Design review of the part built by this model. Coordinates are the model's own, in mm. Face numbers are marked on the shaded views. Coordinates: 2 decimals unless noted, no trailing zeros. Write each loop counter-clockwise with the first axis right and the second up, starting at its lowest first coordinate (ties: lowest second). Pieces come first, ordered by that corner, then holes. Notation, with made-up numbers: M 85.5,11 L 106.5,11 A27 ccw 106.5,28 Z; hole C 19,-31.75 d7. An arc over 180 degrees is marked long. Return JSON: item names as keys, results as strings. Group by question number.
```python
from build123d import *

# Parameters (mm, degrees)
SKETCH1_W           = 110
SKETCH1_H           = 135
SKETCH1_W_2         = 100
SKETCH1_H_2         = 125
BOSS_EXTRUDE1_DEPTH = 200
SKETCH2_W           = 110
SKETCH2_H           = 135
BOSS_EXTRUDE2_DEPTH = 5
CUT_EXTRUDE1_DEPTH  = 12
FILLET1_R           = 3


with BuildPart() as part:
    # Sketch1 → Boss-Extrude1 (new body)
    with BuildSketch(Plane(origin=(0, 0, 0), x_dir=(1, 0, 0), z_dir=(0, 1, 0))):
        Rectangle(SKETCH1_W, SKETCH1_H)
        Rectangle(SKETCH1_W_2, SKETCH1_H_2, mode=Mode.SUBTRACT)
    extrude(amount=BOSS_EXTRUDE1_DEPTH)

    # Sketch2 → Boss-Extrude2 (add)
    with BuildSketch(Plane(origin=(0, 200, 0), x_dir=(1, 0, 0), z_dir=(0, 1, 0))):
        Rectangle(SKETCH2_W, SKETCH2_H)
    extrude(amount=BOSS_EXTRUDE2_DEPTH)

    # Sketch3 → Cut-Extrude1 (cut)
    with BuildSketch(Plane.XZ):
        with BuildLine():
            ThreePointArc((1.45, -65), (0, -63.55), (-1.45, -65))
            Line((-1.45, -65), (1.45, -65))
        make_face()
        with BuildLine():
            Line((1.45, -65), (-1.45, -65))
            ThreePointArc((-1.45, -65), (0, -66.45), (1.45, -65))
        make_face()
        with BuildLine():
            ThreePointArc((53.95, -65), (53.525304833, -63.974695167), (52.5, -63.55))
            Line((52.5, -63.55), (52.5, -65))
            Line((52.5, -65), (51.05, -65))
            ThreePointArc((51.05, -65), (52.5, -66.45), (53.95, -65))
        make_face()
        with BuildLine():
            Line((52.5, -65), (52.5, -63.55))
            ThreePointArc((52.5, -63.55), (51.474695167, -63.974695167), (51.05, -65))
            Line((51.05, -65), (52.5, -65))
        make_face()
        with BuildLine():
            ThreePointArc((53.95, 0), (53.525304833, 1.025304833), (52.5, 1.45))
            Line((52.5, 1.45), (52.5, -1.45))
            ThreePointArc((52.5, -1.45), (53.525304833, -1.025304833), (53.95, 0))
        make_face()
        with BuildLine():
            Line((52.5, -1.45), (52.5, 1.45))
            ThreePointArc((52.5, 1.45), (51.05, 0), (52.5, -1.45))
        make_face()
        with BuildLine():
            ThreePointArc((53.95, 65), (52.5, 66.45), (51.05, 65))
            Line((51.05, 65), (52.5, 65))
            Line((52.5, 65), (52.5, 63.55))
            ThreePointArc((52.5, 63.55), (53.525304833, 63.974695167), (53.95, 65))
        make_face()
        with BuildLine():
            Line((52.5, 65), (51.05, 65))
            ThreePointArc((51.05, 65), (51.474695167, 63.974695167), (52.5, 63.55))
            Line((52.5, 63.55), (52.5, 65))
        make_face()
        with BuildLine():
            ThreePointArc((1.45, 65), (0, 66.45), (-1.45, 65))
            Line((-1.45, 65), (1.45, 65))
        make_face()
        with BuildLine():
            Line((1.45, 65), (-1.45, 65))
            ThreePointArc((-1.45, 65), (0, 63.55), (1.45, 65))
        make_face()
        with BuildLine():
            Line((-52.5, 63.55), (-52.5, 65))
            Line((-52.5, 65), (-51.05, 65))
            ThreePointArc((-51.05, 65), (-53.525304833, 66.025304833), (-52.5, 63.55))
        make_face()
        with BuildLine():
            Line((-51.05, 65), (-52.5, 65))
            Line((-52.5, 65), (-52.5, 63.55))
            ThreePointArc((-52.5, 63.55), (-51.474695167, 63.974695167), (-51.05, 65))
        make_face()
        with BuildLine():
            ThreePointArc((-51.05, 0), (-51.474695167, 1.025304833), (-52.5, 1.45))
            Line((-52.5, 1.45), (-52.5, -1.45))
            ThreePointArc((-52.5, -1.45), (-51.474695167, -1.025304833), (-51.05, 0))
        make_face()
        with BuildLine():
            Line((-52.5, -1.45), (-52.5, 1.45))
            ThreePointArc((-52.5, 1.45), (-53.95, 0), (-52.5, -1.45))
        make_face()
        with BuildLine():
            ThreePointArc((-51.05, -65), (-51.474695167, -63.974695167), (-52.5, -63.55))
            Line((-52.5, -63.55), (-52.5, -65))
            Line((-52.5, -65), (-51.05, -65))
        make_face()
        with BuildLine():
            Line((-52.5, -65), (-52.5, -63.55))
            ThreePointArc((-52.5, -63.55), (-53.525304833, -66.025304833), (-51.05, -65))
            Line((-51.05, -65), (-52.5, -65))
        make_face()
    extrude(amount=-CUT_EXTRUDE1_DEPTH, mode=Mode.SUBTRACT)

    # Fillet1
    fillet1_edges = [part.edges().sort_by_distance(p)[0] for p in [
        (0, 205, -67.5),
        (-55, 205, 0),
        (0, 205, 67.5),
        (55, 205, 0),
        (-55, 102.5, -67.5),
        (55, 102.5, -67.5),
        (55, 102.5, 67.5),
        (-55, 102.5, 67.5),
    ]]
    fillet(fillet1_edges, radius=FILLET1_R)


solid = part.part
```
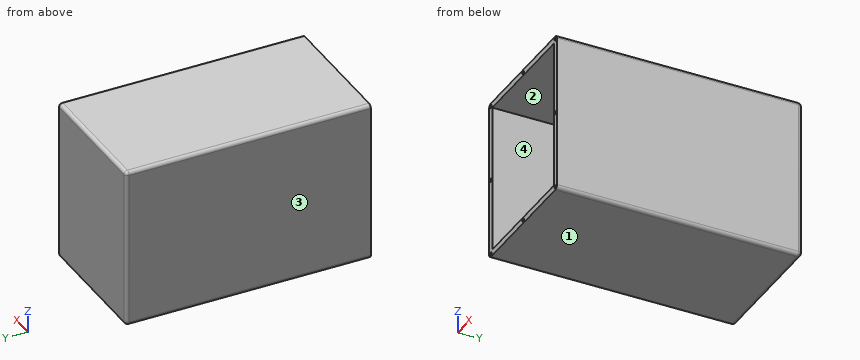
Item 1: Add section A-A (y = 125.5). Write out the cut boundary in (x, z), plus the area to 3 significant figures.
Item 2: The part is to be moulded in two halves that separate along X. For the marked faces 1, 2, 3 and 4, say which applies: pulls with the +X half, pulls with the -X half, needs draft (parallel to the pull), parting line crosses it, or undercut.
Item 3: For line 1 (Z direction, x = -52.5, y = 9); line 2 (X direction, y = 8.5, z = 65); line 3 (Z direction, x = 17, y = 108.5), list the stretches that pass through material, from the lowest coordinate up.
Item 4: Add section C-C (x = 32). Write out the cut boundary in (y, z).
Item 5: Add section B-B (z = 46.5). Write out the cut boundary in (x, y).
Item 6: For pin 1 (1.5 mm diameter, centred on x = -52.5, z = 65.5, fed in from -Y); pin 2 (1.7 mm diameter, centred on x = -52.5, z = -65, fed in from +Y), all flat-tipped, find the tip position at first contact; note any pin that passes through.
Geometry check:
{
 "1": {"outline": "M -55,-64.5 A3 ccw -52,-67.5 L 52,-67.5 A3 ccw 55,-64.5 L 55,64.5 A3 ccw 52,67.5 L -52,67.5 A3 ccw -55,64.5 Z; hole M -50,-62.5 L 50,-62.5 L 50,62.5 L -50,62.5 Z", "area": "2,340 mm^2"},
 "2": {"face 1": "needs draft", "face 2": "undercut", "face 3": "pulls with the -X half", "face 4": "undercut"},
 "3": {"line 1": "-67.46 to -66.45, -63.55 to -1.45, 1.45 to 63.55, 66.45 to 67.46", "line 2": "-54.96 to -53.95, -51.05 to -1.45, 1.45 to 51.05, 53.95 to 54.96", "line 3": "-67.5 to -62.5, 62.5 to 67.5"},
 "4": {"outline": "M 0,-67.5 L 202,-67.5 A3 ccw 205,-64.5 L 205,64.5 A3 ccw 202,67.5 L 0,67.5 L 0,62.5 L 200,62.5 L 200,-62.5 L 0,-62.5 Z"},
 "5": {"outline": "M -55,0 L -50,0 L -50,200 L 50,200 L 50,0 L 55,0 L 55,202 A3 ccw 52,205 L -52,205 A3 ccw -55,202 Z"},
 "6": {"pin 1": "y = 12", "pin 2": "y = 205"}
}
